Source: CAD feature listing. Evaluate the final solid. Frame: model axes, mm. Face numbers are marked on the shaded views. A direction names the side the tool comes from. Coordinates: 2 decimals unless noted, no trailing zeros. Loops run counter-clockwise (first coordinate to the right, second up) from the corner with the lowest first, then second, coordinate; pieces in that order, holes last. Notation, with made-up numbers: (31, 32) -> (48, 32) arc R18 cw to (48, 57) -> close; hole circle Ø11 at (16.25, 80). An arc over 180 degrees is marked (long way). One line per question, with ' | ' between items. Start each with the question number.
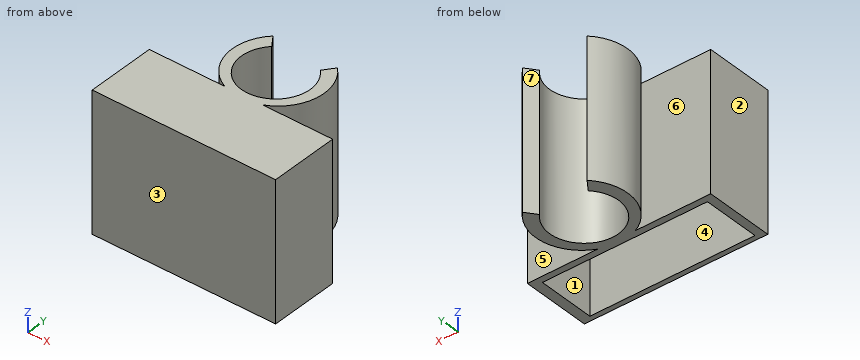
```python
from build123d import *

# Parameters (mm, degrees)
SKETCH1_W           = 80
SKETCH1_H           = 60
BOSS_EXTRUDE2_DEPTH = 30
SKETCH2_W           = 72
SKETCH2_H           = 25
CUT_EXTRUDE1_DEPTH  = 55
BOSS_EXTRUDE3_DEPTH = 60


with BuildPart() as part:
    # Sketch1 → Boss-Extrude2 (new body)
    with BuildSketch(Plane(origin=(0, 0, 0), x_dir=(1, 0, 0), z_dir=(0, 1, 0))):
        with Locations((6.460176991, 17.057522124)):
            Rectangle(SKETCH1_W, SKETCH1_H)
    extrude(amount=BOSS_EXTRUDE2_DEPTH)

    # Sketch2 → Cut-Extrude1 (cut)
    with BuildSketch(Plane(origin=(0, 0, -47.057522124), x_dir=(-1, 0, 0), z_dir=(0, 0, -1))):
        with Locations((-6.207310929, 14.727365754)):
            Rectangle(SKETCH2_W, SKETCH2_H)
    extrude(amount=-CUT_EXTRUDE1_DEPTH, mode=Mode.SUBTRACT)


with BuildPart() as body_2:
    # Sketch3 → Boss-Extrude3 (new body)
    with BuildSketch(Plane(origin=(0, 0, -47.057522124), x_dir=(-1, 0, 0), z_dir=(0, 0, -1))):
        with BuildLine():
            Line((-18.241655929, 57.546020063), (-21.832571653, 62.312614127))
            ThreePointArc((-21.832571653, 62.312614127), (-7.559367185, 28.225064213), (6.451490845, 62.42128158))
            Line((6.451490845, 62.42128158), (2.971534297, 57.569692838))
            ThreePointArc((2.971534297, 57.569692838), (-7.606485249, 31.951270677), (-18.241655929, 57.546020063))
        make_face()
    extrude(amount=-BOSS_EXTRUDE3_DEPTH)

    # Combine1: union part
    add(part.part)


solid = body_2.part
```
(1) Draft query along X for the marked faces 1, 2 and 3. Return one class per face: pulls with the +X half, pulls with the -X half, needs draft (parallel to the pull), parting line crosses it, or undercut.
(2) Ray query, L1, parallel to Y at x = -5, z = -32; L2, parallel to X at y = 16, z = -33; L3, parallel to Y at x = -1, z = 3. Return the intervals inside material, ascending.
(3) Cut plane B-B, the plane x = 30.5. Return the cut outline in (y, z), and give its area (3 significant figures).
(4) Contact query for flat-ended pins moving along their axis: pin 1 Ø3 at (x, z) = (12.5, -41) entering from +Y; pin 2 Ø10 at (x, z) = (-24.5, -12.5) entering from +Y; pin 3 Ø15.5 at (x, z) = (29.5, -18.5) entering from +Y; pin 4 Ø24 at (x, y) = (7.62, 46.95) entering from -Z. Output: stop coordinate, or through.
(5) Cut plane C-C, the plane z = 9. Return the cut outline in (x, y).
(6) Cut plane A-A, the plane z = -18. Return the cut outline in (x, y).
(7) Access query for the marked faces 4, 5, 6 and 7. Directions: +Z, -Z, +X, -X, +Y, -Y. A direction counts if a zero-diameter tool reaches every point of the face in a straight line with its end or side. Return the directions, or none.
(8) Cut plane D-D, the plane y = 24. Return the cut outline in (x, z), and give its area (3 significant figures).
Here are the results:
1) face 1: undercut | face 2: pulls with the -X half | face 3: needs draft
2) L1: y = 0 to 2.23, 27.23 to 30, 32.72 to 38.85, 55.05 to 60.4 | L2: x = -33.54 to -29.79, 42.21 to 46.46 | L3: y = 0 to 2.23, 27.23 to 30, 30.19 to 34.68
3) outline: (0, -47.06) -> (2.23, -47.06) -> (2.23, 7.94) -> (27.23, 7.94) -> (27.23, -47.06) -> (30, -47.06) -> (30, 12.94) -> (0, 12.94) -> close | area: 425 mm2
4) pin 1: stops at y = 33.37 | pin 2: stops at y = 30 | pin 3: stops at y = 62.31 | pin 4: passes through
5) outline: (-33.54, 0) -> (46.46, 0) -> (46.46, 30) -> (15.87, 30) arc R20 ccw to (21.83, 62.31) -> (18.24, 57.55) arc R15 cw (long way) to (-2.97, 57.57) -> (-6.45, 62.42) arc R20 ccw to (-0.6, 30) -> (-33.54, 30) -> close
6) outline: (-33.54, 0) -> (46.46, 0) -> (46.46, 30) -> (15.87, 30) arc R20 ccw to (21.83, 62.31) -> (18.24, 57.55) arc R15 cw (long way) to (-2.97, 57.57) -> (-6.45, 62.42) arc R20 ccw to (-0.6, 30) -> (-33.54, 30) -> close; hole (-29.79, 2.23) -> (42.21, 2.23) -> (42.21, 27.23) -> (-29.79, 27.23) -> close
7) face 4: -Z | face 5: +Z, -Z, +X | face 6: +Z, -Z, -X | face 7: +Z, -Z, +Y
8) outline: (-33.54, -47.06) -> (-29.79, -47.06) -> (-29.79, 7.94) -> (42.21, 7.94) -> (42.21, -47.06) -> (46.46, -47.06) -> (46.46, 12.94) -> (-33.54, 12.94) -> close | area: 840 mm2
